For this review, use the dimensioned drawing (mm, ordinates from the lowest corner) and the shaded views. Coordinates: 2 decimals unless noted, no trailing zeros. Loops run counter-clockwise (first coordinate to the right, second up) from the corner with the lowest first, then second, coordinate; pieces in that order, holes last. Notation, with made-up numbers: M 44.25,-19.5 L 77.25,-19.5 A21 ccw 77.25,11.5 Z; hole C 4.25,-35.75 d5. An arc over 180 degrees is marked long. Use CSV: the item, a comma, the result in double quotes. Start each with the question number.
1. Add section D-D, the plane z = 0.7. State how many separate pieces and enclosed holes the cut face has, then the cut area to 4 significant figures.
2. Add section B-B, the plane y = 177.8. Write out the cut boundary in (x, z) (1 decimal).
3. Add section C-C, the plane y = 38.1. Write out the cut boundary in (x, z) (1 decimal).
4. Clearance check with a flat-ended pin moving along its axis: P1, Ø5, axis at x = 12.7, y = 177.8, coming from the -Z side. State where the tip first meets the part, or that it passes through.
5. For L1, parallel to X at y = 139.5, z = 1.8 (1 decimal); L2, parallel to Y at x = 54.5, z = 2.15; L3, parallel to X at y = 160.5, z = 2.9 (1 decimal), list the stretches that pass through material, from the lowest coordinate up.
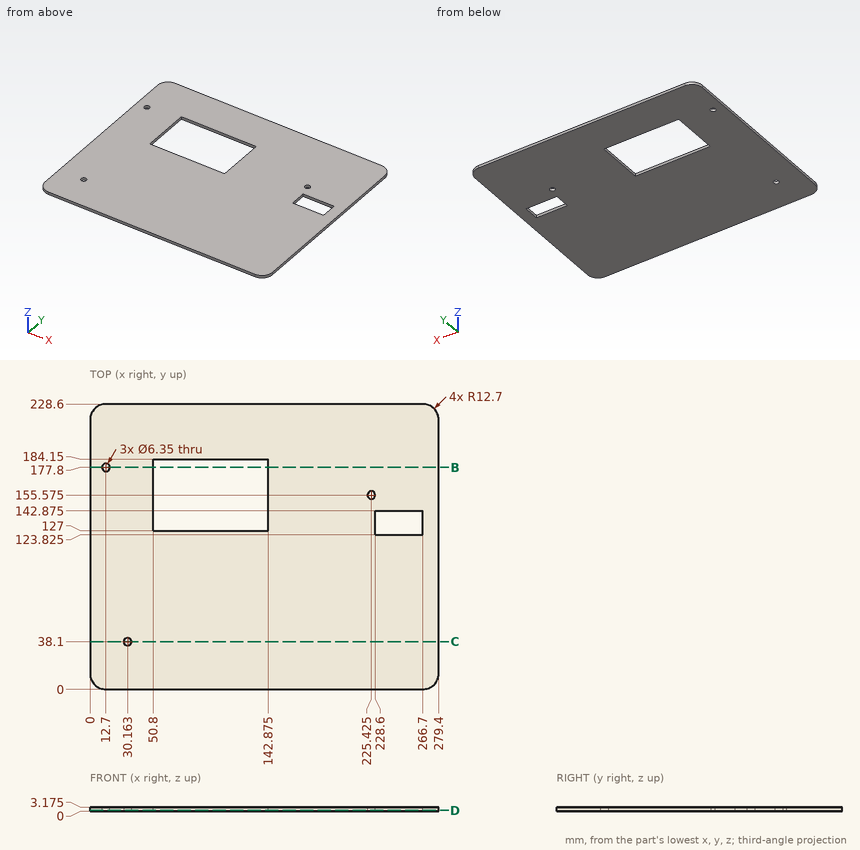
Computed:
1,separate pieces,"1"
1,enclosed holes,"5"
1,area,"57,650 mm^2"
2,outline,"M 0,0 L 9.5,0 L 9.5,3.2 L 0,3.2 Z; M 15.9,0 L 50.8,0 L 50.8,3.2 L 15.9,3.2 Z; M 142.9,0 L 279.4,0 L 279.4,3.2 L 142.9,3.2 Z"
3,outline,"M 0,0 L 27,0 L 27,3.2 L 0,3.2 Z; M 33.3,0 L 279.4,0 L 279.4,3.2 L 33.3,3.2 Z"
4,P1,"passes through"
5,L1,"x = 0 to 50.8, 142.9 to 228.6, 266.7 to 279.4"
5,L2,"y = 0 to 127, 184.15 to 228.6"
5,L3,"x = 0 to 50.8, 142.9 to 279.4"
